```python
from build123d import *

# Parameters (mm, degrees)
SKETCH1_W           = 560
SKETCH1_H           = 75
BOSS_EXTRUDE1_DEPTH = 3
SKETCH2_W           = 3
SKETCH2_H           = 10
CUT_EXTRUDE1_DEPTH  = 3
SKETCH3_W           = 3
SKETCH3_H           = 20
SKETCH3_H_2         = 15
CUT_EXTRUDE2_DEPTH  = 3
SKETCH4_W           = 80
SKETCH4_H           = 3
CUT_EXTRUDE3_DEPTH  = 3


with BuildPart() as part:
    # Sketch1 → Boss-Extrude1 (new body)
    with BuildSketch(Plane.XY):
        with Locations((47.655062333, 176.988975695)):
            Rectangle(SKETCH1_W, SKETCH1_H)
    extrude(amount=BOSS_EXTRUDE1_DEPTH)

    # Sketch2 → Cut-Extrude1 (cut)
    with BuildSketch(Plane.XY.offset(3)):
        with Locations((326.155062333, 189.488975695)):
            Rectangle(SKETCH2_W, SKETCH2_H)
        with Locations((326.155062333, 164.488975695)):
            Rectangle(SKETCH2_W, SKETCH2_H)
    extrude(amount=-CUT_EXTRUDE1_DEPTH, mode=Mode.SUBTRACT)

    # Sketch3 → Cut-Extrude2 (cut)
    with BuildSketch(Plane.XY.offset(3)):
        with Locations((-230.844937667, 204.488975695)):
            Rectangle(SKETCH3_W, SKETCH3_H)
        with Locations((-230.844937667, 149.488975695)):
            Rectangle(SKETCH3_W, SKETCH3_H)
        with Locations((-230.844937667, 176.988975695)):
            Rectangle(SKETCH3_W, SKETCH3_H_2)
    extrude(amount=-CUT_EXTRUDE2_DEPTH, mode=Mode.SUBTRACT)

    # Sketch4 → Cut-Extrude3 (cut)
    with BuildSketch(Plane.XY.offset(3)):
        with Locations((47.655062333, 212.988975695)):
            Rectangle(SKETCH4_W, SKETCH4_H)
    extrude(amount=-CUT_EXTRUDE3_DEPTH, mode=Mode.SUBTRACT)


solid = part.part
```
Here's how the part is built. I have some questions about the finished solid (model axes, mm). Give positions to 0.01 mm unless a question says otherwise; leave off trailing zeros. Loops run counter-clockwise (first coordinate to the right, second up) from the corner with the lowest first, then second, coordinate; pieces in that order, holes last. Notation, with made-up numbers: (74.25, 43) -> (118.25, 43) arc R8 ccw to (118.25, 48) -> close; hole circle Ø1 at (75, 32). An arc over 180 degrees is marked (long way). Use one line per item in the form item = value. Start each with the question number.
1) Imagine slicing it at A-A (x = 16.5). Please give me the cut outline in (y, z).
2) For P1, Ø0.9, axis at x = -230.5, z = 1, coming from the +Y side; P2, Ø1.5, axis at y = 202, z = 1, coming from the -X side; P3, Ø0.9, axis at x = -231, z = 1, coming from the -Y side, each with a flat end and sliding along its axis, tell me the tip position at first contact or that it passes through.
3) Please list where these lines run through material, in increasing order: line 1 along X through (y, z) = (207.5, 0.6); line 2 along X through (y, z) = (194, 2.2); line 3 along Y through (x, z) = (65.5, 1.9).
Check values:
q1.outline = (139.49, 0) -> (211.49, 0) -> (211.49, 3) -> (139.49, 3) -> close
q2.P1 = 194.49
q2.P2 = -229.34
q2.P3 = 159.49
q3.line_1 = -229.34 to 327.66
q3.line_2 = -232.34 to 324.66
q3.line_3 = 139.49 to 211.49
